Read the model definition and answer for the solid it produces. Units are mm, in the model's axes. A direction names the side the tool comes from. Give positions to 0.01 mm unless a question says otherwise; leave off trailing zeros. Order: outer loops, then holes, each group sorted by start corner. A loop starts at its lowest first (then second) coordinate and runs counter-clockwise, first axis right, second up. Notation, with made-up numbers: (-22, 16.5) - (4, 16.5) arc R34 cw to (4, 55.5) - close; hole circle Ø7 at (88.5, 37). An arc over 180 degrees is marked (long way). Write each question's results on one line, items separated by ' | '. Start each with the question number.
Q1. Find section C-C on z = 17. Give the vertices of the cut face in (x, y).
Q2. A tool of negligible diameter and unlimited length cuts with its end or side. For faces 1 (the face through (42.5, 0, 5)), 2 (the face through (24, -41.64, 12)), 3 (the face through (-20.5, -42, 8)), 4 (the face through (-27.5, -42, 8)), from which of +Z, -Z, +X, -X, +Y, -Y can it reach the whole face along a straight path? Write none if from no direction.
Q3. Find section A-A on x = -24. Give the vertices of the cut face in (y, z), and give its area (3 significant figures).
Q4. Find section D-D on y = 10. Give the vertices of the cut face in (x, z), and give its area (4 significant figures).
Q5. For a pull along X with two mould halves and no side action, classify faces 5 (the face through (-4, -29, 7)), 6 (the face through (23.792, -43.612, 15.414)), 7 (the face through (-47.5, 0, 3)), 8 (the face through (47.5, 0, 3)) as +X half, -X half, draft (parallel to the pull), parting line (faces both ways), or undercut.
Q6. Find section B-B on z = 4.75. Give the vertices of the cut face in (x, y), and give its area (3 significant figures).
Q7. Find the intervals of material crossed by line 1 along Y through (x, z) = (26, 4.75); line 2 along Z through (x, y) = (24, -42); line 3 along Y through (x, z) = (-14.5, 3.75), in increasing order. Write a range as from..to.
Q8. Flat-ended cylindrical pins translate along their axes: P1, Ø2, axis at x = 22.5, z = 10, coming from the +Y side; P2, Ø10.5, axis at y = -39.5, z = 13.5, coming from the -X side; P3, Ø3, axis at x = -6, y = -24, coming from the +Z side. Find the tip coordinate at first contact, or state that the pin passes through.
from build123d import *

# Parameters (mm, degrees)
SKETCH1_W           = 85
SKETCH1_H           = 55.6
BOSS_EXTRUDE1_DEPTH = 3.5
SKETCH1_4_W         = 95
SKETCH1_4_H         = 65.6
SKETCH1_4_W_2       = 85
SKETCH1_4_H_2       = 55.6
BOSS_EXTRUDE2_DEPTH = 7
SKETCH1_5_W         = 7
SKETCH1_5_H         = 8.84
BOSS_EXTRUDE3_DEPTH = 3.5
SKETCH1_6_W         = 7
SKETCH1_6_H         = 4
BOSS_EXTRUDE4_DEPTH = 20
CUT_EXTRUDE1_START  = -79.44
SKETCH2_R           = 1.6
CUT_EXTRUDE1_DEPTH  = 80.44


with BuildPart() as part:
    # Sketch1 → Boss-Extrude1 (new body)
    with BuildSketch(Plane.XY):
        Rectangle(SKETCH1_W, SKETCH1_H)
    extrude(amount=BOSS_EXTRUDE1_DEPTH)

    # Sketch1<4> → Boss-Extrude2 (add)
    with BuildSketch(Plane.XY):
        Rectangle(SKETCH1_4_W, SKETCH1_4_H)
        Rectangle(SKETCH1_4_W_2, SKETCH1_4_H_2, mode=Mode.SUBTRACT)
    extrude(amount=BOSS_EXTRUDE2_DEPTH)

    # Sketch1<5> → Boss-Extrude3 (add)
    with BuildSketch(Plane.XY):
        with Locations((-24, -37.22)):
            Rectangle(SKETCH1_5_W, SKETCH1_5_H)
        with Locations((24, -37.22)):
            Rectangle(SKETCH1_5_W, SKETCH1_5_H)
    extrude(amount=BOSS_EXTRUDE3_DEPTH)

    # Sketch1<6> → Boss-Extrude4 (add)
    with BuildSketch(Plane.XY):
        with Locations((-24, -43.64)):
            Rectangle(SKETCH1_6_W, SKETCH1_6_H)
        with Locations((24, -43.64)):
            Rectangle(SKETCH1_6_W, SKETCH1_6_H)
    extrude(amount=BOSS_EXTRUDE4_DEPTH)

    # Sketch2 → Cut-Extrude1 (cut)
    with BuildSketch(Plane(origin=(0, -45.64, 0), x_dir=(-1, 0, 0), z_dir=(0, -1, 0)).offset(CUT_EXTRUDE1_START)):
        with Locations((24, -17)):
            Circle(SKETCH2_R)
    cut_extrude1 = extrude(amount=CUT_EXTRUDE1_DEPTH, mode=Mode.SUBTRACT)

    # Mirror1: Cut-Extrude1 across plane
    add(cut_extrude1.mirror(Plane(origin=(0, 0, 0), x_dir=(0, 0, 1), z_dir=(1, 0, 0))), mode=Mode.SUBTRACT)


solid = part.part
Working result:
1) outline: (-27.5, -45.64) - (-25.6, -45.64) - (-25.6, -41.64) - (-27.5, -41.64) - close; (-22.4, -45.64) - (-20.5, -45.64) - (-20.5, -41.64) - (-22.4, -41.64) - close; (20.5, -45.64) - (22.4, -45.64) - (22.4, -41.64) - (20.5, -41.64) - close; (25.6, -45.64) - (27.5, -45.64) - (27.5, -41.64) - (25.6, -41.64) - close
2) face 1: +Z | face 2: +Z, +X, -X | face 3: +Z, -Z, -Y | face 4: +Z, -Z, -X, -Y
3) outline: (-45.64, 0) - (32.8, 0) - (32.8, 7) - (27.8, 7) - (27.8, 3.5) - (-27.8, 3.5) - (-27.8, 7) - (-32.8, 7) - (-32.8, 3.5) - (-41.64, 3.5) - (-41.64, 15.4) - (-45.64, 15.4) - close; (-45.64, 18.6) - (-41.64, 18.6) - (-41.64, 20) - (-45.64, 20) - close | area: 363 mm²
4) outline: (-47.5, 0) - (47.5, 0) - (47.5, 7) - (42.5, 7) - (42.5, 3.5) - (-42.5, 3.5) - (-42.5, 7) - (-47.5, 7) - close | area: 367.5 mm²
5) face 5: draft | face 6: undercut | face 7: -X half | face 8: +X half
6) outline: (-47.5, -32.8) - (47.5, -32.8) - (47.5, 32.8) - (-47.5, 32.8) - close; (-27.5, -45.64) - (-20.5, -45.64) - (-20.5, -41.64) - (-27.5, -41.64) - close; (20.5, -45.64) - (27.5, -45.64) - (27.5, -41.64) - (20.5, -41.64) - close; hole (-42.5, -27.8) - (42.5, -27.8) - (42.5, 27.8) - (-42.5, 27.8) - close | area: 1,560 mm²
7) line 1: -45.64..-41.64, -32.8..-27.8, 27.8..32.8 | line 2: 0..15.4, 18.6..20 | line 3: -32.8..-27.8, 27.8..32.8
8) P1: y = -41.64 | P2: x = -27.5 | P3: z = 3.5
